The listing builds one solid part. Answer for the finished solid, in the listing's coordinates (mm). Face numbers are marked on the shaded views. Give positions to 0.01 mm unless a question says otherwise; leave off trailing zeros. Write each loop counter-clockwise with the first axis right and the second up, starting at its lowest first coordinate (ties: lowest second). Pieces come first, ordered by that corner, then holes. Notation, with made-up numbers: (66, 83.5) - (94, 83.5) arc R7 ccw to (94, 91.5) - close; hole circle Ø11 at (14, 21). An arc over 180 degrees is marked (long way). One line per question, with ' | ' between items. Start each with the question number.
1. Find the intervals of material crossed by L1, parallel to X at y = 32.5, z = 12.75; L2, parallel to X at y = 39, z = 20; L3, parallel to Y at x = -35, z = 8.25, in increasing order. Write a range as from..to.
2. Given P1, Ø8, axis at x = -9.5, z = 3.5, coming from the -Y side; P2, Ø5, axis at x = -20, z = 16, coming from the +Y side; P3, Ø4, axis at y = -3, z = 19.5, coming from the -X side, each flat-ended and moving along its own axis, determine where each tip first touches the part or whether it passes through.
3. The mould has two halves that part along X. Classify the marked faces 1, 2 and 3: +X half, -X half, draft (parallel to the pull), parting line (faces both ways), or undercut.
4. A cutting plane is placed at A-A (y = 16.5). Determine the outline of the cut face in (x, z), then the cut area to 3 significant figures.
5. A cutting plane is placed at B-B (x = -7). Determine the outline of the cut face in (y, z).
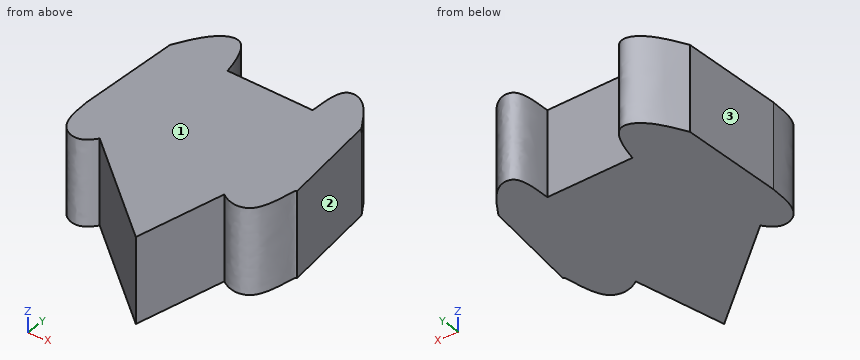
```python
from build123d import *

# Parameters (mm, degrees)
F1_DEPTH = 25


with BuildPart() as f1:
    # F0 (on Top) → F1 (new body)
    with BuildSketch(Plane.XY):
        with BuildLine():
            Line((-18.293430627, 0), (-37.4506600201, 31.5296053886))
            Line((-37.4506600201, 31.5296053886), (-38.6348702013, 0))
            Line((-38.6348702013, 0), (-26.8903197752, -10.3558365563))
            add(Edge.make_bspline(
                [(-26.8903197752, -10.3558365563), (-25.0138511487, -7.7621292657), (-23.3868603398, -3.8810646329), (-21.7598695308, 0)],
                knots=[0.7369926577, 0.7369926577, 0.7369926577, 0.7369926577, 1, 1, 1, 1], degree=3))
            Line((-21.7598695308, 0), (-18.293430627, 0))
        make_face()
        with BuildLine():
            add(Edge.make_bspline(
                [(-37.4506600201, 31.5296053886), (-35.315109491, 35.4914243796), (-31.6617104803, 42.2691172437), (-22.7549071417, 44.5389864619), (-19.8868391117, 31.3424591503), (-19.9717812594, 30.9867953724), (-19.9835542589, 30.937500298)],
                knots=[0, 0, 0, 0, 0.3534616592, 0.6046855171, 0.9452093296, 1, 1, 1, 1], degree=3))
            Line((-37.4506600201, 31.5296053886), (-18.293430627, 0))
            Line((-18.293430627, 0), (-8.7769662755, 0))
            Line((-8.7769662755, 0), (-19.9534838268, 30.9361488185))
            Line((-19.9534838268, 30.9361488185), (-19.9835542589, 30.937500298))
        make_face()
        with BuildLine():
            Line((-26.8903197752, -10.3558365563), (-38.6348702013, 0))
            add(Edge.make_bspline(
                [(-38.6348702013, 0), (-38.4419358813, -4.256929632), (-38.1024093928, -11.748289226), (-30.8831549051, -14.5997468242), (-27.8644585489, -11.7023183486), (-26.8903197752, -10.3558365563)],
                knots=[0, 0, 0, 0, 0.3412066145, 0.6004565887, 0.7369926577, 0.7369926577, 0.7369926577, 0.7369926577], degree=3))
        make_face()
        Polygon((5.1809218712, -38.6348702013), (-18.293430627, 0), (-21.7598695308, 0), align=None)
        Polygon((-8.7769662755, 0), (-18.293430627, 0), (5.1809218712, -38.6348702013), align=None)
        with BuildLine():
            Line((6.3651325181, 29.7532901168), (-19.9534838268, 30.9361488185))
            Line((-19.9534838268, 30.9361488185), (-8.7769662755, 0))
            Line((-8.7769662755, 0), (5.1809218712, 0))
            add(Edge.make_bspline(
                [(5.1809218712, 0), (5.3907033267, -0.660354955), (5.6004847821, -1.32070991), (5.8157272261, -1.9748633921)],
                knots=[0, 0, 0, 0, 0.0490741852, 0.0490741852, 0.0490741852, 0.0490741852], degree=3))
            Line((5.8157272261, -1.9748633921), (6.3651325181, 29.7532901168))
        make_face()
        with BuildLine():
            add(Edge.make_bspline(
                [(-26.8903197752, -10.3558365563), (-25.0138511487, -7.7621292657), (-23.3868603398, -3.8810646329), (-21.7598695308, 0)],
                knots=[0.7369926577, 0.7369926577, 0.7369926577, 0.7369926577, 1, 1, 1, 1], degree=3))
            Line((-26.8903197752, -10.3558365563), (5.1809218712, -38.6348702013))
            Line((5.1809218712, -38.6348702013), (-21.7598695308, 0))
        make_face()
        Polygon((5.1809218712, 0), (-8.7769662755, 0), (5.1809218712, -38.6348702013), align=None)
        with BuildLine():
            Line((5.1809218712, 0), (5.1809218712, -38.6348702013))
            Line((5.1809218712, -38.6348702013), (5.8157272261, -1.9748633921))
            add(Edge.make_bspline(
                [(5.1809218712, 0), (5.3907033267, -0.660354955), (5.6004847821, -1.32070991), (5.8157272261, -1.9748633921)],
                knots=[0, 0, 0, 0, 0.0490741852, 0.0490741852, 0.0490741852, 0.0490741852], degree=3))
        make_face()
        with BuildLine():
            Line((5.8157272261, -1.9748633921), (5.1809218712, -38.6348702013))
            Line((5.1809218712, -38.6348702013), (11.1034761376, -11.4607974057))
            add(Edge.make_bspline(
                [(5.8157272261, -1.9748633921), (7.0525840803, -5.7338535017), (8.4697652594, -9.288068156), (11.1034761376, -11.4607974057)],
                knots=[0.0490741852, 0.0490741852, 0.0490741852, 0.0490741852, 0.3310712728, 0.3310712728, 0.3310712728, 0.3310712728], degree=3))
        make_face()
        with BuildLine():
            add(Edge.make_bspline(
                [(6.3651325181, 29.7532901168), (6.3947430451, 34.2918495311), (6.4439782834, 41.8383904762), (14.1496668788, 40.8069928969), (17.9473376206, 34.5091520104), (20.2796068043, 30.6414496154)],
                knots=[0, 0, 0, 0, 0.3679740058, 0.6118529357, 1, 1, 1, 1], degree=3))
            Line((6.3651325181, 29.7532901168), (5.8157272261, -1.9748633921))
            add(Edge.make_bspline(
                [(5.8157272261, -1.9748633921), (7.0525840803, -5.7338535017), (8.4697652594, -9.288068156), (11.1034761376, -11.4607974057)],
                knots=[0.0490741852, 0.0490741852, 0.0490741852, 0.0490741852, 0.3310712728, 0.3310712728, 0.3310712728, 0.3310712728], degree=3))
            Line((11.1034761376, -11.4607974057), (20.2796068043, 30.6414496154))
        make_face()
        with BuildLine():
            Line((20.2796068043, 30.6414496154), (11.1034761376, -11.4607974057))
            add(Edge.make_bspline(
                [(11.1034761376, -11.4607974057), (11.2000080599, -11.5404332278), (13.9535287523, -13.7221274774), (22.647914545, -15.1627090559), (23.2770923169, 0.4801138246), (24.0272593597, 0.0569857777), (24.1282898933, 0)],
                knots=[0.3310712728, 0.3310712728, 0.3310712728, 0.3310712728, 0.3414071533, 0.6209883528, 0.9489557035, 1, 1, 1, 1], degree=3))
            Line((24.1282898933, 0), (20.2796068043, 30.6414496154))
        make_face()
    extrude(amount=F1_DEPTH)


solid = f1.part
```
Determined:
1) L1: -36.93..-20.22, 6.4..19.15 | L2: -32.91..-22.29, 7.25..14.3 | L3: -12.36..35.91
2) P1: y = -29.22 | P2: y = 39.45 | P3: x = -38.59
3) face 1: draft | face 2: +X half | face 3: -X half
4) outline: (-38.02, 0) - (22.06, 0) - (22.06, 25) - (-38.02, 25) - close | area: 1,500 mm2
5) outline: (-27.89, 0) - (30.35, 0) - (30.35, 25) - (-27.89, 25) - close
